The model under review builds one solid part; all positions refer to its coordinate system, in mm. Face numbers are marked on the shaded views. A direction names the side the tool comes from. Give positions to 0.01 mm unless a question says otherwise; leave off trailing zeros. Loops run counter-clockwise (first coordinate to the right, second up) from the corner with the lowest first, then second, coordinate; pieces in that order, holes last. Notation, with made-up numbers: M 19.25,83 L 53.25,83 A26 cw 53.25,106 Z; hole C -36.75,81 d7. An arc over 180 degrees is marked long. Write item = value, one per line. Start each with the question number.
1. For pin 1 (1.2 mm diameter, centred on x = 13.5, y = 6, fed in from +Z); pin 2 (1 mm diameter, centred on x = 17, z = 4.5, fed in from +Y); pin 3 (1.5 mm diameter, centred on x = 17.5, z = 18.5, fed in from -Y), all flat-tipped, find the tip position at first contact; note any pin that passes through.
2. We need section A-A on y = 6. Give the boundary of the cut face in (x, z).
3. For the marked faces 1 and 2, list the 3-axis set-ups (+Z, -Z, +X, -X, +Y, -Y) from which the entire face can be reached by the end or side of a thin tool; tool diameter is ignored.
4. We need section C-C on z = 29. Give the boundary of the cut face in (x, y).
5. We need section D-D on y = 2.5. Give the boundary of the cut face in (x, z).
6. Wall thickness on line 1 along Z through (x, y) = (3.5, 10.5); line 2 along Z through (x, y) = (12.5, 4.5); line 3 along X through (y, z) = (1.75, 14): over which ranges is each line inside the solid? List them lowest first. Write a range as from..to.
7. We need section B-B on x = 9.25. Give the boundary of the cut face in (y, z), then the cut area to 3 significant figures.
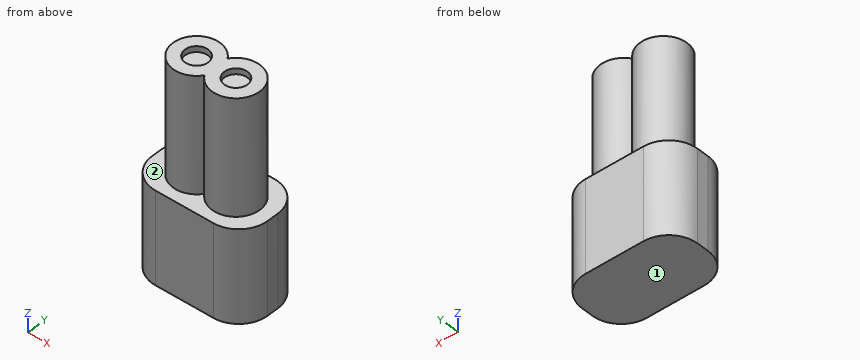
from build123d import *

# Parameters (mm, degrees)
EXTRUDE_1_DEPTH     = 16
EXTRUDE_3_DEPTH     = 20
SKETCH_4_R          = 2
CUT_EXTRUDE_1_DEPTH = 1


with BuildPart() as part:
    # ｽｹｯﾁ1 → ﾎﾞｽ - 押し出し1 (new body)
    with BuildSketch(Plane.XY):
        with BuildLine():
            Line((5, 0), (15, 0))
            ThreePointArc((15, 0), (18.535533906, 1.464466094), (20, 5))
            Line((20, 5), (20, 7))
            ThreePointArc((20, 7), (18.535533906, 10.535533906), (15, 12))
            Line((15, 12), (5, 12))
            ThreePointArc((5, 12), (1.464466094, 10.535533906), (0, 7))
            Line((0, 7), (0, 5))
            ThreePointArc((0, 5), (1.464466094, 1.464466094), (5, 0))
        make_face()
    extrude(amount=EXTRUDE_1_DEPTH)

    # ｽｹｯﾁ3 → ﾎﾞｽ - 押し出し3 (add)
    with BuildSketch(Plane.XY.offset(16)):
        with BuildLine():
            ThreePointArc((10.178530878, 3.727869439), (17.760027495, 6), (10.178530878, 8.272130561))
            ThreePointArc((10.178530878, 8.272130561), (2.735636676, 6), (10.178530878, 3.727869439))
        make_face()
    extrude(amount=EXTRUDE_3_DEPTH)

    # ｽｹｯﾁ4 → ｶｯﾄ - 押し出し1 (cut)
    with BuildSketch(Plane.XY.offset(36)):
        with Locations((6.803896263, 6)):
            Circle(SKETCH_4_R)
        with Locations((13.628807012, 6)):
            Circle(SKETCH_4_R)
    extrude(amount=-CUT_EXTRUDE_1_DEPTH, mode=Mode.SUBTRACT)


solid = part.part
Final values:
q1.pin_1 = 35
q1.pin_2 = 11.77
q1.pin_3 = 3.29
q2.outline = M 0,0 L 20,0 L 20,16 L 17.76,16 L 17.76,36 L 15.63,36 L 15.63,35 L 11.63,35 L 11.63,36 L 8.8,36 L 8.8,35 L 4.8,35 L 4.8,36 L 2.74,36 L 2.74,16 L 0,16 Z
q3.face_1 = -Z, +X, -X, +Y, -Y
q3.face_2 = +Z
q4.outline = M 10.18,3.73 A4.13 ccw long 10.18,8.27 A4.07 ccw long Z
q5.outline = M 0.67,0 L 19.33,0 L 19.33,16 L 15.82,16 L 15.82,36 L 11.43,36 L 11.43,16 L 8.88,16 L 8.88,36 L 4.73,36 L 4.73,16 L 0.67,16 Z
q6.line_1 = 0..16
q6.line_2 = 0..35
q6.line_3 = 1.2..18.8
q7.outline = M 0,0 L 12,0 L 12,16 L 9.25,16 L 9.25,36 L 2.75,36 L 2.75,16 L 0,16 Z
q7.area = 322 mm²
